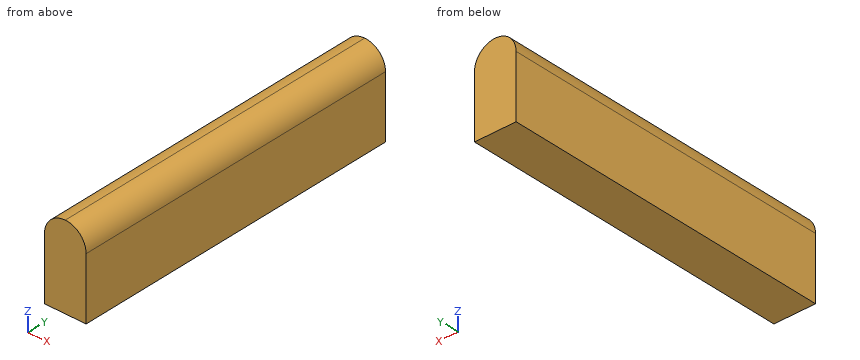
```python
from build123d import *

# Parameters (mm, degrees)
F1_DEPTH = 10
F2_R     = 2.49999
F3_W     = 11.3749653101
F3_H     = 21.1809808388
F4_DEPTH = 25
F5_DEPTH = 25


# Not quite as in the source:
# - a fillet or chamfer is up to 0.001 mm smaller than in the source, because OpenCascade refuses the exact size


with BuildPart() as f1:
    # F0 (on Top) → F1 (new body)
    with BuildSketch(Plane.XY):
        Polygon((-44.6886586582, 25.7738458982), (-44.6886586582, -29.2261541018), (-39.6886586582, -29.2261541018), (-39.6886586582, 20.7738458982), (30.3113413418, 20.7738458982), (30.3113413418, -29.2261541018), (35.3113413418, -29.2261541018), (35.3113413418, 25.7738458982), align=None)
    extrude(amount=F1_DEPTH)

    # F2 (radius 2.5 in the source; OpenCascade refuses exactly that, so slightly less here)
    f2_edges = [f1.edges().sort_by_distance(p)[0] for p in [
        (-44.688659, -1.726154, 10),
        (-39.688659, -4.226154, 10),
        (30.311341, -4.226154, 10),
        (35.311341, -1.726154, 10),
    ]]
    fillet(f2_edges, radius=F2_R)

    # F3 (on Top) → F4 (cut)
    with BuildSketch(Plane.XY):
        Polygon((47.2649559379, 40.0085151196), (-24.1227895021, 40.0085151196), (-24.1227895021, 10.9827276319), (-24.1227895021, -10.1982532069), (-35.4977548122, -10.1982532069), (-35.4977548122, -43.5386821628), (47.2649559379, -43.5386821628), align=None)
        Polygon((-35.4977548122, 10.9827276319), (-35.4977548122, 40.0085151196), (-24.1227895021, 40.0085151196), (-24.1227895021, 54.521407932), (-54.7175332904, 54.521407932), (-54.7175332904, 10.9827276319), align=None)
        with Locations((-29.8102721572, 0.3922372125)):
            Rectangle(F3_W, F3_H)
    extrude(amount=F4_DEPTH, mode=Mode.SUBTRACT)

    # F5 (cut): a face of the model
    f5_faces = [f1.faces().sort_by_distance(p)[0] for p in [
        (-24.1227895021, 23.2738458982, 5),
    ]]
    extrude(f5_faces, amount=-F5_DEPTH, mode=Mode.SUBTRACT)


solid = f1.part
```
Geometry check sheet. Reference: the model listing, model coordinates, mm. Coordinates: 2 decimals unless noted, no trailing zeros. Loops run counter-clockwise (first coordinate to the right, second up) from the corner with the lowest first, then second, coordinate; pieces in that order, holes last.
Item 1: Thickness scan on line 1 (Z direction, x = -44.3, y = 8); line 2 (Z direction, x = -42.1, y = 6.5); line 3 (X direction, y = -18, z = 7.75). Record the ranges inside material, lowest first.
Item 2: Sectioned sample at B-B, the plane x = -43.35. Record the boundary of the cut face in (y, z).
Item 3: Go/stop test with a flat-tipped pin: pin 1 Ø1 at (x, y) = (-40.5, -8) entering from +Z. Record where the tip stops, or that it passes through.
Item 4: Sectioned sample at C-C, the plane z = 8.25. Record the boundary of the cut face in (x, y).
Check result:
1. line 1: z = 0 to 8.84
1. line 2: z = 0 to 10
1. line 3: x = -44.68 to -39.7
2. outline: (-29.23, 0) - (10.98, 0) - (10.98, 9.71) - (-29.23, 9.71) - close
3. pin 1: stops at z = 9.7
4. outline: (-44.57, -29.23) - (-39.8, -29.23) - (-39.8, 10.98) - (-44.57, 10.98) - close
